Autodesk Inventor part; units mm, degrees
ref_plane "YZ Plane" through (0, 0, 0) normal (1, 0, 0) x (0, 1, 0)
ref_plane "XZ Plane" through (0, 0, 0) normal (0, 1, 0) x (-1, 0, 0)
ref_plane "XY Plane" through (0, 0, 0) normal (0, 0, 1) x (1, 0, 0)
sketch "Sketch1" plane through (0, 0, 0) normal (0, 0, 1) x (1, 0, 0)
  circle A0 centre (0, 0) radius 5
  circle A1 centre (0, 0) radius 10
  dimension "d0" = 10
  dimension "d1" = 20
extrude "Extrusion1" add sketch "Sketch1" along normal blind 4.5
sketch "Sketch2" plane through (0, 0, 4.5) normal (0, 0, 1) x (1, 0, 0)
  circle A0 centre (0, 0) radius 10
  circle A1 centre (0, 0) radius 9.75
  circle A2 centre (0, 0) radius 5
  circle A3 centre (0, 0) radius 5.25
  dimension "d4" = 19.5
  dimension "d5" = 10
  dimension "d6" = 10.5
extrude "Extrusion2" add sketch "Sketch2" along normal blind 0.25
sketch "Sketch3" plane through (0, 0, 0) normal (0, 0, -1) x (-1, 0, 0)
  circle A0 centre (0, 0) radius 10
  circle A1 centre (0, 0) radius 9.75
  circle A2 centre (0, 0) radius 5
  circle A3 centre (0, 0) radius 5.25
  dimension "d9" = 20
  dimension "d10" = 19.5
  dimension "d11" = 10
  dimension "d12" = 10.5
extrude "Extrusion3" add sketch "Sketch3" along normal blind 0.25
properties part number "bearing" material "Aluminum 6061"
Geometry: final body of the model. Coordinates: model frame, mm. A direction names the side the tool comes from. Round coordinates to 2 decimals unless told otherwise and drop trailing zeros. Write each loop counter-clockwise with the first axis right and the second up, starting at its lowest first coordinate (ties: lowest second). Pieces come first, ordered by that corner, then holes. Notation, with made-up numbers: (75.5, 41) -> (104.5, 41) arc R16 ccw to (104.5, 45) -> close; hole circle Ø3 at (18.5, 9.5). An arc over 180 degrees is marked (long way). Use CSV: the item, a comma, the result in double quotes. Start each with the question number.
Q1. Section A-A (y = 0). Return loops of the section in (x, z).
Q2. First-contact query: pin 1 Ø1 at (x, z) = (-3.5, 1.5) entering from +Y; pin 2 Ø1.5 at (y, z) = (1.5, 1.5) entering from +X; pin 3 Ø1 at (y, z) = (7, 4) entering from -X; pin 4 Ø6 at (x, y) = (-2, -5) entering from -Z. Flat tips, straight axial feed; report the tip coordinate or a pass-through.
Q3. Section C-C (z = 3.45). Return loops of the section in (x, y).
Q4. Line query: L1, parallel to Y at x = 0, z = 4.65; L2, parallel to X at y = 0, z = 4.25. Output: solid intervals per line, ascending.
Q5. Section D-D (x = -8.5). Return loops of the section in (y, z), plus the area to 3 significant figures.
Q6. Reachability of faces 1 (the face through (4, -4, 4.5)), 2 (the face through (4, -4, 0)) from +Z, -Z, +X, -X, +Y, -Y: full face, straight path, thin tool, end or side. Return the list, or none.
Result sheet:
1,outline,"(-10, -0.25) -> (-9.75, -0.25) -> (-9.75, 0) -> (-5.25, 0) -> (-5.25, -0.25) -> (-5, -0.25) -> (-5, 4.75) -> (-5.25, 4.75) -> (-5.25, 4.5) -> (-9.75, 4.5) -> (-9.75, 4.75) -> (-10, 4.75) -> close; (5, -0.25) -> (5.25, -0.25) -> (5.25, 0) -> (9.75, 0) -> (9.75, -0.25) -> (10, -0.25) -> (10, 4.75) -> (9.75, 4.75) -> (9.75, 4.5) -> (5.25, 4.5) -> (5.25, 4.75) -> (5, 4.75) -> close"
2,pin 1,"y = 9.54"
2,pin 2,"x = 9.97"
2,pin 3,"x = -7.6"
2,pin 4,"z = -0.25"
3,outline,"circle Ø20 at (0, 0); hole circle Ø10 at (0, 0)"
4,L1,"-10 to -9.75, -5.25 to -5, 5 to 5.25, 9.75 to 10"
4,L2,"-10 to -5, 5 to 10"
5,outline,"(-5.27, -0.25) -> (-4.78, -0.25) -> (-4.78, 0) -> (4.78, 0) -> (4.78, -0.25) -> (5.27, -0.25) -> (5.27, 4.75) -> (4.78, 4.75) -> (4.78, 4.5) -> (-4.78, 4.5) -> (-4.78, 4.75) -> (-5.27, 4.75) -> close"
5,area,"47.9 mm²"
6,face 1,"+Z"
6,face 2,"-Z"
